CAD build for the part. Positions are in the model's coordinates, mm. A direction names the side the tool comes from. Round coordinates to 2 decimals unless told otherwise and drop trailing zeros. Loops run counter-clockwise (first coordinate to the right, second up) from the corner with the lowest first, then second, coordinate; pieces in that order, holes last.
```python
from build123d import *

# Parameters (mm, degrees)
SKETCH_2_W          = 21
SKETCH_2_H          = 18
EXTRUDE_2_DEPTH     = 5
EXTRUDE_3_DEPTH     = 9
SKETCH_4_W          = 30
SKETCH_4_H          = 1
CUT_EXTRUDE_1_DEPTH = 60.968741858
FILLET_1_R          = 0.5
FILLET_2_R          = 2.5
FILLET_3_R          = 5
CHAMFER_1_SIZE      = 1
SKETCH_5_R          = 1.7
CUT_EXTRUDE_2_DEPTH = 55.398988961
SKETCH_6_W          = 6
SKETCH_6_H          = 1
EXTRUDE_4_DEPTH     = 1


with BuildPart() as part:
    # ｽｹｯﾁ2 → ﾎﾞｽ - 押し出し2 (new body)
    with BuildSketch(Plane(origin=(0, 0, 0), x_dir=(1, 0, 0), z_dir=(0, 1, 0))):
        Rectangle(SKETCH_2_W, SKETCH_2_H)
    extrude(amount=EXTRUDE_2_DEPTH)

    # ｽｹｯﾁ3 → ﾎﾞｽ - 押し出し3 (add)
    with BuildSketch(Plane(origin=(0, -4, 0), x_dir=(-1, 0, 0), z_dir=(0, -1, 0))):
        Polygon((-5.5, 9), (-35.5, 34), (-41.5, 34), (-41.5, 33), (-35.5, 31.5), (-10.5, 4), align=None)
    extrude(amount=-EXTRUDE_3_DEPTH)

    # ｽｹｯﾁ4 → ｶｯﾄ - 押し出し1 (cut, through all)
    with BuildSketch(Plane.XY.offset(9)):
        Polygon((35.5, -1), (10.5, 5), (41.5, 5), (41.5, -1), align=None)
        with Locations((20.5, -3.5)):
            Rectangle(SKETCH_4_W, SKETCH_4_H)
    extrude(amount=-CUT_EXTRUDE_1_DEPTH, mode=Mode.SUBTRACT)

    # ﾌｨﾚｯﾄ1
    fillet_1_edges = [part.edges().sort_by_distance(p)[0] for p in [
        (41.5, -2.5, -33),
    ]]
    fillet(fillet_1_edges, radius=FILLET_1_R)

    # ﾌｨﾚｯﾄ2
    fillet_2_edges = [part.edges().sort_by_distance(p)[0] for p in [
        (8, 0, -6.5),
    ]]
    fillet(fillet_2_edges, radius=FILLET_2_R)

    # ﾌｨﾚｯﾄ3
    fillet_3_edges = [part.edges().sort_by_distance(p)[0] for p in [
        (-10.5, 2.5, -9),
    ]]
    fillet(fillet_3_edges, radius=FILLET_3_R)

    # 面取り1
    chamfer_1_edges = [part.edges().sort_by_distance(p)[0] for p in [
        (10.5, 2.5, 9),
        (-10.5, 2.5, 9),
    ]]
    chamfer(chamfer_1_edges, length=CHAMFER_1_SIZE)

    # ｽｹｯﾁ5 → ｶｯﾄ - 押し出し2 (cut, through all)
    with BuildSketch(Plane(origin=(0, 5, 0), x_dir=(1, 0, 0), z_dir=(0, 1, 0))):
        with Locations(Location((6, 0, 0), (0, 0, 270))):
            Circle(SKETCH_5_R)
        with Locations(Location((-6, 0, 0), (0, 0, 270))):
            Circle(SKETCH_5_R)
    extrude(amount=-CUT_EXTRUDE_2_DEPTH, mode=Mode.SUBTRACT)

    # ｽｹｯﾁ6 → ﾎﾞｽ - 押し出し4 (add)
    with BuildSketch(Plane(origin=(0, 0, -34), x_dir=(-1, 0, 0), z_dir=(0, 0, -1))):
        with Locations((-38.5, -3.5)):
            Rectangle(SKETCH_6_W, SKETCH_6_H)
    extrude(amount=EXTRUDE_4_DEPTH)


solid = part.part
```
Item 1: 3-axis set-ups, long thin cutter, end or side, ignore diameter. For faces 1 (the flat face through (0, 0, 0)), 2 (the flat face through (38, -1, -33)), 3 (the flat face through (41.5, -2.9, -33.8)), 4 (the flat face through (38, -2, -34)): which of +Z, -Z, +X, -X, +Y, -Y reach the whole face in a straight line?
Answers follow:
face 1: +Z, -X, -Y
face 2: +Z, -Z, +X, +Y
face 3: +Z, -Z, +X, +Y, -Y
face 4: -Z, +X, -X, +Y
Item 2: Cut at B-B, the plane x = 31. Give the cut face in (y, z), plus the area to 3 significant figures.
Answers follow:
outline: (-3, -30.25) - (0.08, -30.25) - (0.08, -26.55) - (-3, -26.55) - close
area: 11.4 mm2
Item 3: Cut at C-C, the plane z = 3. Give the cut face in (x, y), plus the area to 3 significant figures.
Answers follow:
outline: (-10.5, 0) - (10.5, 0) - (10.5, 5) - (-10.5, 5) - close
area: 105 mm2
Item 4: Two-plate mould, pull along X, no slides. Class faces 5 (the cylindrical face through (4.34, 2.54, -0.37)), 6 (the flat face through (38.3, -2.5, -32.2)), 7 (the flat face through (8, -2.8, -6.5)): released by +X, released by -X, zero draft, split by the parting line, or undercut.
Answers follow:
face 5: undercut
face 6: released by +X
face 7: released by -X
Item 5: Probe line 1 (X direction, y = 3.1, z = 0); line 2 (Y direction, x = 3.5, z = 2); line 3 (Z direction, x = 0, y = 2.5). List the from-to ranges inside material, lowest first.
Answers follow:
line 1: x = -10.5 to -7.7, -4.3 to 4.3, 7.7 to 10.5
line 2: y = 0 to 5
line 3: z = -9 to 9
Item 6: Cut at A-A, the plane y = 1.25. Give the cut face in (x, z) (1 decimal), plus the area to 3 significant figures.
Answers follow:
outline: (-10.5, -4) arc R5 ccw to (-5.5, -9) - (5.5, -9) - (26.1, -26.2) - (26.1, -21.2) - (10.5, -4) - (10.5, 8) - (9.5, 9) - (-9.5, 9) - (-10.5, 8) - close; hole circle Ø3.4 at (-6, 0); hole circle Ø3.4 at (6, 0)
area: 475 mm2
Item 7: Flat gauge pins, fed straight in: P1, Ø3.5, axis at x = 0, y = 3, coming from the -Z side; P2, Ø0.5, axis at x = 37.5, z = -34.5, coming from the +Y side; P3, Ø0.6, axis at x = 39, y = -2, coming from the -Z side. Where does each tip first touch, or does it go through?
Answers follow:
P1: stops at z = -9
P2: stops at y = -3
P3: stops at z = -34
